Design review of the part shown in the three views and the two pictorial views. Dimensions are in mm from the part's minimum x, y and z. Coordinates: 2 decimals unless noted, no trailing zeros. Loops run counter-clockwise (first coordinate to the right, second up) from the corner with the lowest first, then second, coordinate; pieces in that order, holes last. Notation, with made-up numbers: (38.5, -40) -> (81.5, -40) arc R14 cw to (81.5, -29) -> close; hole circle Ø7 at (5, 61). An arc over 180 degrees is marked (long way). Answer in a Markdown table with one row per item.
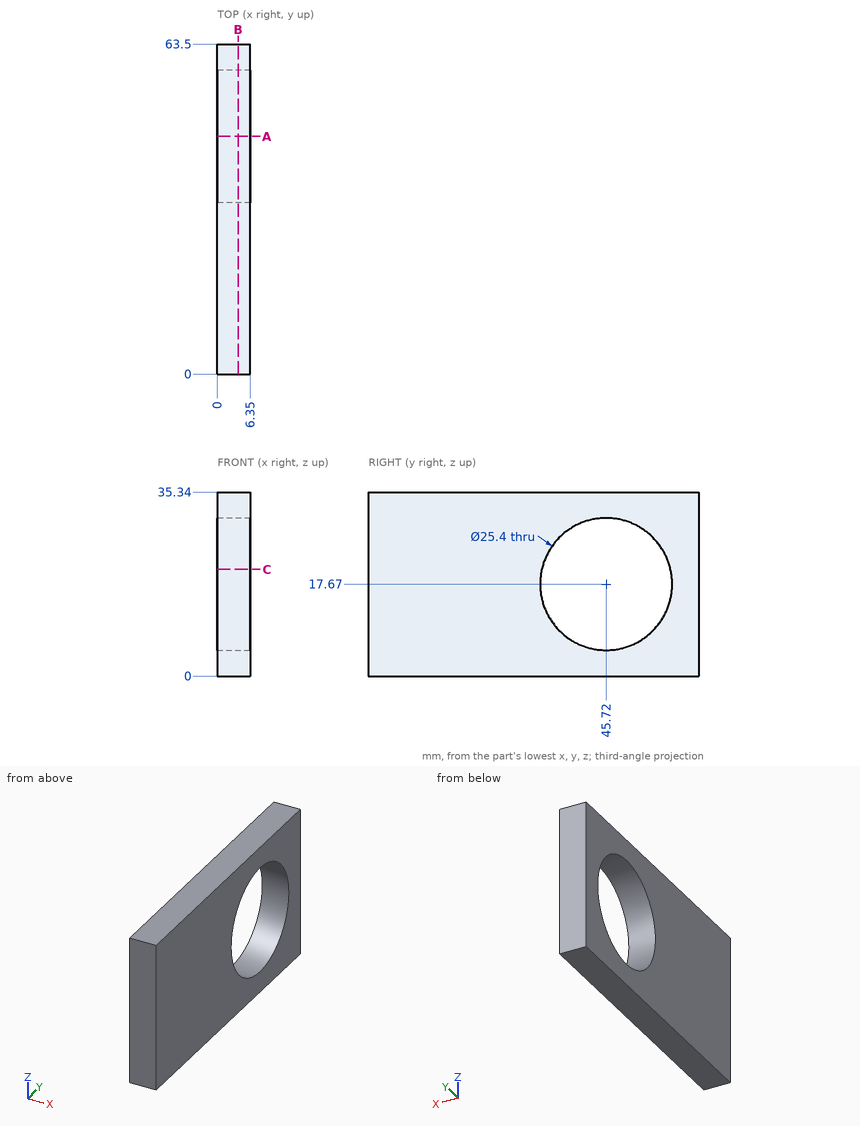
Item 1: Take a section at B-B, the plane x = 4. State the section outline as (y, z) points.
Worked answers:
| item | result |
|---|---|
| outline | (0, 0) -> (63.5, 0) -> (63.5, 35.34) -> (0, 35.34) -> close; hole circle Ø25.4 at (45.72, 17.67) |
Item 2: Insertion check: pin 1 (1 mm diameter, centred on x = 5, y = 8.5, fed in from -Z). The pin has a flat end and moves straight along its axis. Give the tip position at first contact, or say it passes through.
Worked answers:
| item | result |
|---|---|
| pin 1 | z = 0 |
Item 3: For L1, parallel to Z at x = 1.25, y = 37 (1 decimal); L2, parallel to Y at x = 4.75, z = 26.5; L3, parallel to Y at x = 6, z = 18.5, list the stretches that pass through material, from the lowest coordinate up.
Worked answers:
| item | result |
|---|---|
| L1 | 0 to 8.4, 26.9 to 35.3 |
| L2 | 0 to 36.59, 54.85 to 63.5 |
| L3 | 0 to 33.05, 58.39 to 63.5 |
Item 4: Take a section at A-A, the plane y = 45.72. State the section outline as (x, z) points.
Worked answers:
| item | result |
|---|---|
| outline | (0, 0) -> (6.35, 0) -> (6.35, 4.97) -> (0, 4.97) -> close; (0, 30.37) -> (6.35, 30.37) -> (6.35, 35.34) -> (0, 35.34) -> close |
Item 5: Take a section at C-C, the plane z = 20.5. State the section outline as (x, y) points.
Worked answers:
| item | result |
|---|---|
| outline | (0, 0) -> (6.35, 0) -> (6.35, 33.34) -> (0, 33.34) -> close; (0, 58.1) -> (6.35, 58.1) -> (6.35, 63.5) -> (0, 63.5) -> close |
